Autodesk Inventor part; units mm, degrees
ref_plane "YZ Plane" through (0, 0, 0) normal (1, 0, 0) x (0, 1, 0)
ref_plane "XZ Plane" through (0, 0, 0) normal (0, 1, 0) x (-1, 0, 0)
ref_plane "XY Plane" through (0, 0, 0) normal (0, 0, 1) x (1, 0, 0)
sketch "Skizze1" plane through (0, 0, 0) normal (0, 1, 0) x (-1, 0, 0)
  line L0 (127.3199, 0) -> (-102.7808, 0) construction
  line L1 (0, 142.2638) -> (0, -235.5235) construction
  line L2 (100, 50) -> (100, 0)
  line L3 (70, 50) -> (0, 50)
  line L4 (0, 0) -> (100, 0)
  line L5 (0, 50) -> (0, 0)
  line L6 (100, 50) -> (100, 170)
  line L7 (100, 170) -> (70, 170)
  line L8 (70, 170) -> (70, 50)
  circle A0 centre (95, 46) radius 1.7
  dimension "d10" = 100
  dimension "d12" = 30
  dimension "d13" = 170
  dimension "d14" = 50
  dimension "d22" = 5
  dimension "d23" = 4
  dimension "d26" = 3.4
extrude "Extrusion1" add sketch "Skizze1" along normal blind 5
ref_plane "Arbeitsebene1" through (0, 0, 50) normal (1, 0, 0) x (0, 1, 0)
ref_plane "Arbeitsebene2" through (0, 5, 0) normal (0, 0, -1) x (-1, 0, 0)
mirror "Spiegeln1" about plane through (0, 5, 0) normal (0, 0, -1) of "Extrusion1"
pattern_circular "Runde Anordnung1" count 2 over 360 about axis through (0, 5, 0) along (0, -1, 0) of "Extrusion1"
mirror "Spiegeln2" about plane through (0, 0, 50) normal (1, 0, 0) of "Extrusion1"
mirror "Spiegeln3" about plane through (0, 5, 0) normal (0, 0, -1) of "Extrusion1"
sketch "Skizze2" plane through (0, 0, 0) normal (0, -1, 0) x (1, 0, 0)
  line L0 (-100, 170) -> (-100, -170) construction
  line L1 (-100, 170) -> (-70, 170) construction
  line L2 (-100, 140) -> (-70, 140)
  line L3 (-70, 170) -> (-70, 50)
  circle A0 centre (-85, 155) radius 5
  point P0 (0, 0)
  dimension "d28" = 30
  dimension "d29" = 15
  dimension "d31" = 10
extrude "Extrusion3" cut sketch "Skizze2" against normal blind 10
properties part number "Chassis-1"
Geometry check sheet. Reference: the model listing, model coordinates, mm. Round coordinates to 2 decimals unless told otherwise and drop trailing zeros. Write each loop counter-clockwise with the first axis right and the second up, starting at its lowest first coordinate (ties: lowest second). Pieces come first, ordered by that corner, then holes. Notation, with made-up numbers: (7, 35) -> (30, 35) arc R25 cw to (30, 71) -> close; hole circle Ø10 at (85, 47). An arc over 180 degrees is marked (long way). Put each result on its own line as item: value.
1) Release check for a two-part mould opening along Z. For faces 1 (the face through (1, 5, 2)), 2 (the face through (-80.381, 2.465, 153.085)) record: pulls with the +Z half, pulls with the -Z half, needs draft (parallel to the pull), parting line crosses it, or undercut.
Recorded:
face 1: needs draft
face 2: undercut
2) Cross-section at A-A, the plane z = 155. Enter the section's corners in (x, y), plus the area to 3 significant figures.
Recorded:
outline: (-100, 0) -> (-90, 0) -> (-90, 5) -> (-100, 5) -> close; (-80, 0) -> (-70, 0) -> (-70, 5) -> (-80, 5) -> close; (70, 0) -> (100, 0) -> (100, 5) -> (70, 5) -> close
area: 250 mm2
3) Depth check by flat-ended pin: P1, Ø1.5, axis at x = -72.5, z = -18, coming from the -Y side. Enter the tip coordinate at first touch or a pass-through.
Recorded:
P1: stops at y = 0
4) Cross-section at D-D, the plane z = 89.5. Enter the section's corners in (x, y), plus the area to 3 significant figures.
Recorded:
outline: (-100, 0) -> (-70, 0) -> (-70, 5) -> (-100, 5) -> close; (70, 0) -> (100, 0) -> (100, 5) -> (70, 5) -> close
area: 300 mm2
5) Cross-section at C-C, the plane x = -85. Enter the section's corners in (y, z).
Recorded:
outline: (0, -170) -> (5, -170) -> (5, 150) -> (0, 150) -> close; (0, 160) -> (5, 160) -> (5, 170) -> (0, 170) -> close
6) Cross-section at B-B, the plane y = 3.2. Enter the section's corners in (x, z).
Recorded:
outline: (-100, -170) -> (-70, -170) -> (-70, -50) -> (70, -50) -> (70, -170) -> (100, -170) -> (100, 170) -> (70, 170) -> (70, 50) -> (-70, 50) -> (-70, 170) -> (-100, 170) -> close; hole circle Ø3.4 at (-95, -46); hole circle Ø3.4 at (-95, 46); hole circle Ø10 at (-85, 155); hole circle Ø3.4 at (95, -46); hole circle Ø3.4 at (95, 46)
7) Thickness scan on probe 1 along X at (y, z) = (2.75, -46); probe 2 along Z at (x, y) = (-95, 2.7); probe 3 along X at (y, z) = (1.25, -65.5). Record the ranges inside material, lowest first. Write a range as from..to.
Recorded:
probe 1: x = -100..-96.7, -93.3..93.3, 96.7..100
probe 2: z = -170..-47.7, -44.3..44.3, 47.7..170
probe 3: x = -100..-70, 70..100
